```python
from build123d import *

# Parameters (mm, degrees)
BOSS_EXTRUDE1_DEPTH = 3
BOSS_EXTRUDE2_DEPTH = 11
SKETCH3_W           = 28
SKETCH3_H           = 50
SKETCH3_W_2         = 54
SKETCH3_H_2         = 12
BOSS_EXTRUDE3_DEPTH = 4
SKETCH4_W           = 15
SKETCH4_H           = 10
BOSS_EXTRUDE4_DEPTH = 17


with BuildPart() as part:
    # Model → Boss-Extrude1 (new body)
    with BuildSketch(Plane.XY):
        with BuildLine():
            ThreePointArc((38.829215393, -80.915724874), (0, 89.75), (-38.829215393, -80.915724874))
            add(Edge.make_bspline(
                [(38.829215393, -80.915724874), (12.943071798, -72.694758375), (-12.943071798, -72.694758375), (-38.829215393, -80.915724874)],
                knots=[0, 0, 0, 0, 1, 1, 1, 1], degree=3))
        make_face()
        Polygon((-20.854851634, -43.482268632), (-37.546710486, -60.174127484), (-32.596963018, -65.123874952), (-43.203564736, -75.73047667), (-75.73047667, -43.203564736), (-65.123874952, -32.596963018), (-60.174127484, -37.546710486), (-43.482268632, -20.854851634), align=None, mode=Mode.SUBTRACT)
        Polygon((43.482268632, -20.854851634), (60.174127484, -37.546710486), (65.123874952, -32.596963018), (75.73047667, -43.203564736), (43.203564736, -75.73047667), (32.596963018, -65.123874952), (37.546710486, -60.174127484), (20.854851634, -43.482268632), align=None, mode=Mode.SUBTRACT)
        Polygon((20.854851634, 43.482268632), (37.546710486, 60.174127484), (32.596963018, 65.123874952), (43.203564736, 75.73047667), (75.73047667, 43.203564736), (65.123874952, 32.596963018), (60.174127484, 37.546710486), (43.482268632, 20.854851634), align=None, mode=Mode.SUBTRACT)
        Polygon((-43.482268632, 20.854851634), (-60.174127484, 37.546710486), (-65.123874952, 32.596963018), (-75.73047667, 43.203564736), (-43.203564736, 75.73047667), (-32.596963018, 65.123874952), (-37.546710486, 60.174127484), (-20.854851634, 43.482268632), align=None, mode=Mode.SUBTRACT)
    extrude(amount=BOSS_EXTRUDE1_DEPTH)

    # Sketch2 → Boss-Extrude2 (add)
    with BuildSketch(Plane.XY.offset(3)):
        with BuildLine():
            Line((-38.829215393, -80.915724874), (-38.601028715, -79.915724874))
            ThreePointArc((-38.601028715, -79.915724874), (0, 88.75), (38.601028715, -79.915724874))
            Line((38.601028715, -79.915724874), (38.829215393, -80.915724874))
            ThreePointArc((38.829215393, -80.915724874), (0, 89.75), (-38.829215393, -80.915724874))
        make_face()
    extrude(amount=BOSS_EXTRUDE2_DEPTH)

    # Sketch3 → Boss-Extrude3 (add)
    with BuildSketch(Plane.XY.offset(3)):
        with Locations((0, -34.75)):
            Rectangle(SKETCH3_W, SKETCH3_H)
        with Locations((0, -65.75)):
            Rectangle(SKETCH3_W_2, SKETCH3_H_2)
    extrude(amount=BOSS_EXTRUDE3_DEPTH)

    # Sketch4 → Boss-Extrude4 (add)
    with BuildSketch(Plane.XY.offset(7)):
        with Locations((0, -16.75)):
            Rectangle(SKETCH4_W, SKETCH4_H)
    extrude(amount=BOSS_EXTRUDE4_DEPTH)


solid = part.part
```
The model under review builds one solid part; all positions refer to its coordinate system, in mm. A direction names the side the tool comes from. Give positions to 0.01 mm unless a question says otherwise; leave off trailing zeros. Write each loop counter-clockwise with the first axis right and the second up, starting at its lowest first coordinate (ties: lowest second). Pieces come first, ordered by that corner, then holes. Notation, with made-up numbers: (57.25, -30) - (107.25, -30) arc R29 ccw to (107.25, 5) - close; hole circle Ø3 at (-38.5, 72). An arc over 180 degrees is marked (long way). Answer in a Markdown table with one row per item. Add a question column.
1. We need section B-B on y = -30. Write out the cut boundary in (x, z), then the cut area to 3 significant figures.
2. Wall thickness on line 1 along X through (y, z) = (-37, 6); line 2 along X through (y, z) = (0, 11); line 3 along X through (y, z) = (-70, 1.75): over which ranges is each line inside the solid? List them lowest first. Write a range as [from, to].
3. We need section D-D on z = 22. Write out the cut boundary in (x, y), then the cut area to 3 significant figures.
4. Insertion check: P1, Ø3, axis at x = 60, y = -15.5, coming from the +Z side; P2, Ø8, axis at x = 66.5, z = 4.5, coming from the +Y side; P3, Ø2, axis at y = -63.5, z = 6, coming from the -X side. Each pin has a flat end and moves straight along its axis. Give the tip position at first contact, or say it passes through.
5. We need section A-A on z = 9.5. Write out the cut boundary in (x, y), then the cut area to 3 significant figures.
6. We need section C-C on y = 0. Write out the cut boundary in (x, z).
7. Tool access review of faces 1 (the flat face through (0, -21.75, 15)), 2 (the flat face through (29.08, 51.71, 1.48)): name each direction out of +Z, -Z, +X, -X, +Y, -Y from which nothing blocks a thin tool from reaching the whole face with its end or side.
8. Draft analysis for pull direction X (two halves, no side actions). For faces 3 (the flat face through (-1, 6, 0)), 4 (the cylindrical face through (3.384, 89.686, 6.902)), 5 (the flat face through (-7.5, -17, 15)), state which applies: +X half, -X half, draft (parallel to the pull), parting line (faces both ways), or undercut.
Ans:
| question | item | result |
|---|---|---|
| 1 | outline | (-84.59, 0) - (-52.63, 0) - (-52.63, 3) - (-83.53, 3) - (-83.53, 14) - (-84.59, 14) - close; (-34.34, 0) - (34.34, 0) - (34.34, 3) - (14, 3) - (14, 7) - (-14, 7) - (-14, 3) - (-34.34, 3) - close; (52.63, 0) - (84.59, 0) - (84.59, 14) - (83.53, 14) - (83.53, 3) - (52.63, 3) - close |
| 1 | area | 533 mm^2 |
| 2 | line 1 | x = [-81.77, -80.67], [-14, 14], [80.67, 81.77] |
| 2 | line 2 | x = [-89.75, -88.75], [88.75, 89.75] |
| 2 | line 3 | x = [-56.17, -48.93], [-37.47, 37.47], [48.93, 56.17] |
| 3 | outline | (-7.5, -21.75) - (7.5, -21.75) - (7.5, -11.75) - (-7.5, -11.75) - close |
| 3 | area | 150 mm^2 |
| 4 | P1 | stops at z = 3 |
| 4 | P2 | stops at y = 64.41 |
| 4 | P3 | stops at x = -64.41 |
| 5 | outline | (-38.83, -80.92) - (-38.6, -79.92) arc R88.75 cw (long way) to (38.6, -79.92) - (38.83, -80.92) arc R89.75 ccw (long way) to start; (-7.5, -21.75) - (7.5, -21.75) - (7.5, -11.75) - (-7.5, -11.75) - close |
| 5 | area | 631 mm^2 |
| 6 | outline | (-89.75, 0) - (89.75, 0) - (89.75, 14) - (88.75, 14) - (88.75, 3) - (-88.75, 3) - (-88.75, 14) - (-89.75, 14) - close |
| 7 | face 1 | +Z, -Y |
| 7 | face 2 | +Z, -Z |
| 8 | face 3 | draft |
| 8 | face 4 | parting line |
| 8 | face 5 | undercut |
